Solid Edge part; units mm, degrees
sketch "Sketch1" plane through (0, 0, 0) normal (0, -1, 0) x (1, 0, 0)
  line L0 (16, 20) -> (-44, 20)
  line L1 (-44, 20) -> (-44, -20)
  line L2 (-44, -20) -> (16, -20)
  line L3 (16, -20) -> (16, 20)
  dimension "D1" = 16
  dimension "D2" = 16
extrude "Protrusion1" add sketch "Sketch1" against normal blind 24.5
sketch "Sketch2" plane through (-14, 24.5, 0) normal (0, 1, 0) x (0, 0, 1)
  line L0 (-16, -24.5) -> (16, -24.5)
  line L1 (16, -24.5) -> (16, 25.5)
  line L2 (16, 25.5) -> (-16, 25.5)
  line L3 (-16, 25.5) -> (-16, -24.5)
  dimension "D1" = 16
  dimension "D2" = 16
extrude "VaciadoExtruido_2" cut sketch "Sketch2" against normal blind 10
sketch "Sketch3" plane through (-13.5, 14.5, 0) normal (0, 1, 0) x (0, 0, 1)
  line L0 (-10.5, -19.5) -> (10.5, -19.5)
  line L1 (10.5, -19.5) -> (10.5, 13.5)
  line L2 (10.5, 13.5) -> (-10.5, 13.5)
  line L3 (-10.5, 13.5) -> (-10.5, -19.5)
  dimension "D1" = 10.5
  dimension "D2" = 10.5
extrude "VaciadoExtruido_3" cut sketch "Sketch3" against normal blind 3
sketch "Sketch4" plane through (-14, 0, 0) normal (0, -1, 0) x (0, 0, -1)
  line L0 (-20, 30) -> (-50, 30)
  line L1 (-50, 30) -> (-50, -30)
  line L2 (-50, -30) -> (-20, -30)
  dimension "D1" = 20
extrude "Protrusion2" add sketch "Sketch4" against normal up to vertex (12.25 mm away) material side at (15.95, 0, 35)
hole "Agujero_1" at (-25, 12.25, 0) direction (0, -1, 0) diameter 7 end through all
hole "Hole1" at (-2.5, 12.25, 30) direction (0, -1, 0) diameter 7 end through all
hole "Hole2" at (-22.5, 12.25, 30) direction (0, -1, 0) diameter 7 end through all
sketch "Sketch5" plane through (-44, 12.25, 15) normal (-1, 0, 0) x (0, 0, -1)
  line L0 (-35, 9.25) -> (35, 9.25)
  line L1 (35, 9.25) -> (35, -12.25)
  line L2 (35, -12.25) -> (-35, -12.25)
  line L3 (-35, -12.25) -> (-35, 9.25)
extrude "Cutout1" cut sketch "Sketch5" against normal through all
sketch "Sketch6" plane through (-14, 0, 15) normal (0, -1, 0) x (-1, 0, 0)
  line L0 (30, -35) -> (30, 35)
  line L1 (-30, 35) -> (30, 35)
  line L2 (-30, 35) -> (-30, -35)
  line L3 (-35, -35) -> (-30, -35)
  line L4 (-35, 40) -> (-35, -35)
  line L5 (-35, 40) -> (35, 40)
  line L6 (35, -35) -> (35, 40)
  line L7 (30, -35) -> (35, -35)
  dimension "D1" = 30
  dimension "D2" = 35
  dimension "D3" = 35
  dimension "D4" = 30
extrude "Protrusion3" add sketch "Sketch6" against normal up to vertex (3 mm away)
hole "Agujero_4" at (11, 0, -15) direction (0, 1, 0) diameter 7 end through all countersink diameter 13.71 countersink angle 90
hole "Hole3" at (-39, 0, -15) direction (0, 1, 0) diameter 7 end through all countersink diameter 13.71 countersink angle 90
hole "Hole4" at (-12.5, 0, 43) direction (0, 1, 0) diameter 7 end through all countersink diameter 13.71 countersink angle 90
hole "Hole5" at (-25, 0, 0) direction (0, 1, 0) diameter 7 end through all countersink diameter 13.71 countersink angle 90
sketch "Sketch7" plane through (-14, 0, 12.5) normal (0, -1, 0) x (-1, 0, 0)
  line L0 (-35, 52.5) -> (35, 52.5)
  line L1 (35, 52.5) -> (35, 37.5)
  line L2 (-35, 37.5) -> (35, 37.5)
  line L3 (-35, 37.5) -> (-35, 52.5)
extrude "Protrusion4" add sketch "Sketch7" against normal up to vertex (3 mm away)
hole "Agujero_12" at (-25, 0, -30) direction (0, 1, 0) diameter 4.134 end up to next thread major 5 thread length 2
hole "Hole6" at (0, 0, -30) direction (0, 1, 0) diameter 4.134 end up to next thread major 5 thread length 2
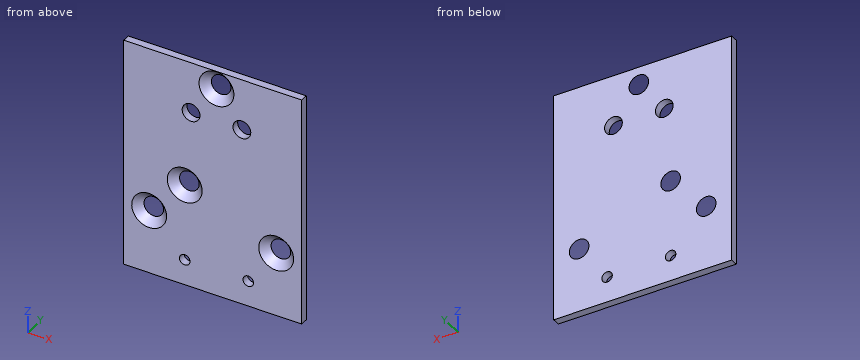
For this review, take the finished solid that the model builds, in its own axes (mm). Round coordinates to 2 decimals unless told otherwise and drop trailing zeros. Write each loop counter-clockwise with the first axis right and the second up, starting at its lowest first coordinate (ties: lowest second). Pieces come first, ordered by that corner, then holes. Notation, with made-up numbers: M -21.75,18 L -6.75,18 A8 ccw -6.75,25 Z; hole C -36,78.25 d9. An arc over 180 degrees is marked long. Write item = value, one per line. Start each with the question number.
(1) For line 1 along X through (y, z) = (2, -30); line 2 along X through (y, z) = (1.9, 30); line 3 along Z through (x, y) = (-24, 2.65), list the stretches that pass through material, from the lowest coordinate up.
(2) Clearance check with a flat-ended pin moving along its axis: pin 1 Ø6.5 at (x, z) = (-2.5, 30) entering from -Y. State where the tip first meets the part, or that it passes through.
(3) We need section A-A (z = 30). Give the boundary of the cut face in (x, y).
(4) We need section C-C (y = 2.25). Give the number of separate pieces and of enclosed holes in the cut face, then the cut area to 3 significant figures.
(5) We need section B-B (x = 0). Give the boundary of the cut face in (y, z).
(6) We need section D-D (x = -25). Give the boundary of the cut face in (y, z) (3 decimals).
Results found:
q1.line_1 = -49 to -27.07, -22.93 to -2.07, 2.07 to 21
q1.line_2 = -49 to -26, -19 to -6, 1 to 21
q1.line_3 = -40 to -31.81, -28.19 to -4.08, 4.08 to 26.84, 33.16 to 50
q2.pin_1 = through
q3.outline = M -49,0 L -26,0 L -26,3 L -49,3 Z; M -19,0 L -6,0 L -6,3 L -19,3 Z; M 1,0 L 21,0 L 21,3 L 1,3 Z
q4.separate_pieces = 1
q4.enclosed_holes = 8
q4.area = 5,930 mm²
q5.outline = M 0,-40 L 3,-40 L 3,-32.07 L 0,-32.07 Z; M 0,-27.93 L 3,-27.93 L 3,27.55 L 0,27.55 Z; M 0,32.45 L 3,32.45 L 3,50 L 0,50 Z
q6.outline = M 0,-40 L 3,-40 L 3,-32.067 L 0,-32.067 Z; M 0,-27.933 L 3,-27.933 L 3,-3.855 L 0,-6.855 Z; M 0,6.855 L 3,3.855 L 3,27.551 L 0,27.551 Z; M 0,32.449 L 3,32.449 L 3,50 L 0,50 Z
